Autodesk Inventor part; units mm, degrees
ref_plane "YZ Plane" through (0, 0, 0) normal (1, 0, 0) x (0, 1, 0)
ref_plane "XZ Plane" through (0, 0, 0) normal (0, 1, 0) x (-1, 0, 0)
ref_plane "XY Plane" through (0, 0, 0) normal (0, 0, 1) x (1, 0, 0)
sketch "Sketch1" plane through (0, 0, 0) normal (0, 0, 1) x (1, 0, 0)
  line L0 (-2.05, 2.05) -> (2.05, 2.05)
  line L1 (2.05, 2.05) -> (2.05, -2.05)
  line L2 (2.05, -2.05) -> (-2.05, -2.05)
  line L3 (-2.05, -2.05) -> (-2.05, 2.05)
  line L4 (0, 2.05) -> (0, -2.05) construction
  line L5 (0, 7.5) -> (-15.55, 7.5)
  line L6 (-15.55, 7.5) -> (-15.55, 6)
  line L7 (-15.55, 6) -> (-3.55, 6)
  line L8 (-3.55, 6) -> (-3.55, -6)
  line L9 (-3.55, -6) -> (-15.55, -6)
  line L10 (-15.55, -6) -> (-15.55, -7.5)
  line L11 (-15.55, -7.5) -> (-0.55, -7.5)
  line L12 (-2.05, 0) -> (2.05, 0) construction
  line L13 (0, 7.5) -> (15.55, 7.5)
  line L14 (15.55, 7.5) -> (15.55, 6)
  line L15 (15.55, 6) -> (3.55, 6)
  line L16 (3.55, 6) -> (3.55, -6)
  line L17 (3.55, -6) -> (15.55, -6)
  line L18 (15.55, -6) -> (15.55, -7.5)
  line L19 (15.55, -7.5) -> (-0.55, -7.5)
  line L20 (-2.05, 2.05) -> (2.05, -2.05) construction
  line L21 (2.05, 2.05) -> (-2.05, -2.05) construction
  line L22 (0, 7.5) -> (0, 2.05) construction
  line L23 (-3.55, 6) -> (-3.55, 7.5)
  line L24 (-3.55, -6) -> (-3.55, -7.5)
  line L25 (3.55, 6) -> (3.55, 7.5)
  line L26 (3.55, -6) -> (3.55, -7.5)
  point P0 (0, 0)
  point P1 (0, 0)
  point P2 (0, 0)
  dimension "d3" = 4.1
  dimension "d4" = 4.1
  dimension "d5" = 12
  dimension "d6" = 1.5
  dimension "d7" = 1.5
  dimension "d8" = 5.45
  dimension "d9" = 5.45
  dimension "d10" = 1.5
  dimension "d11" = 12
  dimension "d37" = 15
extrude "Extrusion1" add sketch "Sketch1" along normal blind 10 contours L13 L25 L16 L26 L19 L11 L24 L8 L23 L5
sketch "Sketch5" plane through (0, 0, 10) normal (0, 0, 1) x (1, 0, 0)
  line L0 (6, 19.5) -> (7.5, 19.5)
  line L1 (7.5, 19.5) -> (7.5, 7.5)
  line L2 (7.5, 7.5) -> (6, 7.5)
  line L3 (6, 7.5) -> (6, 19.5)
  line L4 (3.55, 7.5) -> (-3.55, 7.5)
  line L5 (3.55, -7.5) -> (3.55, 7.5)
  line L6 (0, 0) -> (0, 23.4065) construction
  point P0 (15.55, 7.5)
  point P1 (-15.55, 7.5)
  point P2 (3.55, -6)
  point P3 (3.55, 6)
  dimension "d41" = 1.5
  dimension "d42" = 12
  dimension "d47" = 6
extrude "Extrusion5" add sketch "Sketch5" against normal up to surface (10 mm away)
mirror "Mirror1" about plane through (0, 0, 0) normal (1, 0, 0) of "Extrusion5"
sketch "Sketch7" plane through (0, 0, 10) normal (0, 0, 1) x (1, 0, 0)
  line L0 (-7.5, 19.5) -> (-7.5, 7.5)
  line L1 (-7.5, 7.5) -> (7.5, 7.5)
  line L2 (7.5, 7.5) -> (7.5, 6)
  line L3 (7.5, 6) -> (-7.5, 6)
  line L4 (-7.5, 6) -> (-7.5, 7.5)
  line L5 (7.5, 7.5) -> (7.5, 19.5)
  point P0 (0, 0)
  dimension "d53" = 1.5
extrude "Extrusion7" add sketch "Sketch7" against normal up to surface (10 mm away)
fillet "Fillet3" radius 1 4 edges at (-3.55, 6, 5) (3.55, 6, 5) (7.5, 6, 5) (-7.5, 6, 5)
sketch "Sketch8" plane through (0, 0, 10) normal (0, 0, 1) x (1, 0, 0)
  line L0 (-3.55, -3.55) -> (3.55, -3.55)
  line L1 (3.55, -3.55) -> (3.55, -7.5)
  line L2 (3.55, -7.5) -> (-3.55, -7.5)
  line L3 (-3.55, -7.5) -> (-3.55, -3.55)
  line L4 (2.05, -2.05) -> (-2.05, -2.05)
  line L5 (3.55, -7.5) -> (3.55, 5)
  line L6 (-3.55, 5) -> (-3.55, -7.5)
  line L7 (-3.55, -7.5) -> (3.55, -7.5)
  point P0 (0, 0)
  dimension "d57" = 1.5
extrude "Extrusion8" cut sketch "Sketch8" against normal blind 10
fillet "Fillet4" radius 2 4 edges at (-6.75, 19.5, 10) (-6.75, 19.5, 0) (6.75, 19.5, 0) (6.75, 19.5, 10)
fillet "Fillet5" radius 2 2 edges at (3.55, -3.55, 5) (-3.55, -3.55, 5)
equation "\"d7\" = d6"
equation "\"d8\" = d9"
properties part number "fuselage_tail_interface_airfoiled" material "ABS Plastic"
Source: CAD feature listing. Evaluate the final solid. Frame: model axes, mm. A direction names the side the tool comes from. Round coordinates to 2 decimals unless told otherwise and drop trailing zeros. Write each loop counter-clockwise with the first axis right and the second up, starting at its lowest first coordinate (ties: lowest second). Pieces come first, ordered by that corner, then holes. Notation, with made-up numbers: M 28,58.25 L 36,58.25 A20 cw 36,62.25 Z; hole C 69,-28 d3. An arc over 180 degrees is marked long. One line per item, written item: value. Start each with the question number.
Item 1: Pin query (flat end, axial travel): pin 1 (4 mm diameter, centred on y = 3, z = 5.5, fed in from -X); pin 2 (1 mm diameter, centred on x = -2.5, z = 8.5, fed in from +Y); pin 3 (1 mm diameter, centred on y = 5, z = 4.5, fed in from +X). Return the tip coordinate at first contact, or that it passes through.
Item 2: Mould query, pull axis X, two halves, no side actions, for faces 1 (the flat face through (-3.55, 2, 5)), 2 (the flat face through (0, 2.05, 5)), 3 (the cylindrical face through (-6.76, 18.9, 9.43)). Classes: pulls with the +X half, pulls with the -X half, needs draft (parallel to the pull), parting line crosses it, or undercut.
Item 3: Section query C-C (z = 7). Return the cut outline in (x, y).
Item 4: Section query A-A (x = 1.25). Return the cut outline in (y, z), plus the area to 3 significant figures.
Item 5: Set-up query: faces 4 (the cylindrical face through (6.76, 18.93, 9.4)), 5 (the flat face through (0, -2.05, 5)), 6 (the flat face through (3.55, 2, 5)). Return all of +Z, -Z, +X, -X, +Y, -Y with unobstructed straight access to the full face (end or side cutting, diameter ignored); none if empty.
Item 6: Ray query, L1, parallel to Y at x = 0.5, z = 5.25; L2, parallel to X at y = 17.75, z = 5; L3, parallel to X at y = -1.25, z = 7. Return the intervals inside material, ascending. Write a range as from..to.
Item 7: Section query D-D (x = 5.5). Return the cut outline in (y, z).
Item 8: Section query B-B (y = 11.75). Return the cut outline in (x, z).
Result set:
1. pin 1: stops at x = -3.55
1. pin 2: stops at y = 7.5
1. pin 3: stops at x = 3.68
2. face 1: pulls with the -X half
2. face 2: undercut
2. face 3: needs draft
3. outline: M -7.5,7 A1 ccw -6.5,6 L -4.55,6 A1 cw -3.55,5 L -3.55,-1.55 A2 ccw -1.55,-3.55 L 1.55,-3.55 A2 ccw 3.55,-1.55 L 3.55,5 A1 cw 4.55,6 L 6.5,6 A1 ccw 7.5,7 L 7.5,19.5 L 6,19.5 L 6,7.5 L -6,7.5 L -6,19.5 L -7.5,19.5 Z; hole M -2.05,-2.05 L 2.05,-2.05 L 2.05,2.05 L -2.05,2.05 Z
4. outline: M -3.55,0 L -2.05,0 L -2.05,10 L -3.55,10 Z; M 2.05,0 L 7.5,0 L 7.5,10 L 2.05,10 Z
4. area: 69.5 mm²
5. face 4: +Z, +X, -X, +Y
5. face 5: +Z, -Z
5. face 6: +Z, -Z, +X, -Y
6. L1: y = -3.55..-2.05, 2.05..7.5
6. L2: x = -7.5..-6, 6..7.5
6. L3: x = -3.55..-2.05, 2.05..3.55
7. outline: M 6,0 L 7.5,0 L 7.5,10 L 6,10 Z
8. outline: M -7.5,0 L -6,0 L -6,10 L -7.5,10 Z; M 6,0 L 7.5,0 L 7.5,10 L 6,10 Z
